from build123d import *

# Parameters (mm, degrees)
SKETCH_W        = 50
SKETCH_H        = 30
SKETCH_R        = 1.7
PAD_DEPTH       = 30
SKETCH001_W     = 16
SKETCH001_H     = 35
POCKET_DEPTH    = 24
POCKET001_DEPTH = 4
SKETCH003_R     = 2.5
POCKET002_DEPTH = 1.7
SKETCH004_R     = 3.6
POCKET003_DEPTH = 24
POCKET004_DEPTH = 4
SKETCH006_R     = 1.5
POCKET005_DEPTH = 20
FILLET_R        = 4
FILLET001_R     = 4
FILLET002_R     = 4
FILLET003_R     = 4
FILLET004_R     = 1
FILLET005_R     = 1
FILLET006_R     = 1
FILLET007_R     = 1
FILLET008_R     = 1
FILLET009_R     = 1
FILLET010_R     = 1
FILLET011_R     = 1


with BuildPart() as part:
    # Sketch → Pad (new body)
    with BuildSketch(Plane.XY):
        Rectangle(SKETCH_W, SKETCH_H)
        with Locations((18, 10)):
            Circle(SKETCH_R, mode=Mode.SUBTRACT)
        with Locations((18, -10)):
            Circle(SKETCH_R, mode=Mode.SUBTRACT)
        with Locations((-18, -10)):
            Circle(SKETCH_R, mode=Mode.SUBTRACT)
        with Locations((-18, 10)):
            Circle(SKETCH_R, mode=Mode.SUBTRACT)
    extrude(amount=PAD_DEPTH)

    # Sketch001 → Pocket (cut)
    with BuildSketch(Plane.XY.offset(30)):
        with Locations((-10, 0)):
            Rectangle(SKETCH001_W, SKETCH001_H)
        with Locations((10, 0)):
            Rectangle(SKETCH001_W, SKETCH001_H)
    extrude(amount=-POCKET_DEPTH, mode=Mode.SUBTRACT)

    # Sketch002 → Pocket001 (cut)
    with BuildSketch(Plane(origin=(0, 0, 0), x_dir=(1, 0, 0), z_dir=(0, 0, -1))):
        Polygon((-12.309401, 4), (-14.618802, 0), (-12.309401, -4), (-7.690599, -4), (-5.381198, 0), (-7.690599, 4), align=None)
        Polygon((7.690599, 4), (5.381198, 0), (7.690599, -4), (12.309401, -4), (14.618802, 0), (12.309401, 4), align=None)
    extrude(amount=-POCKET001_DEPTH, mode=Mode.SUBTRACT)

    # Sketch003 → Pocket002 (cut)
    with BuildSketch(Plane.XY.offset(6)):
        with Locations((-10, 0)):
            Circle(SKETCH003_R)
        with Locations((10, 0)):
            Circle(SKETCH003_R)
    extrude(amount=-POCKET002_DEPTH, mode=Mode.SUBTRACT)

    # Sketch004 → Pocket003 (cut)
    with BuildSketch(Plane.XY.offset(30)):
        with Locations((-18, 10)):
            Circle(SKETCH004_R)
        with Locations((18, 10)):
            Circle(SKETCH004_R)
        with Locations((-18, -10)):
            Circle(SKETCH004_R)
        with Locations((18.251301, -10.165039)):
            Circle(SKETCH004_R)
    extrude(amount=-POCKET003_DEPTH, mode=Mode.SUBTRACT)

    # Sketch005 → Pocket004 (cut)
    with BuildSketch(Plane.XY.offset(6)):
        Polygon((-19.558846, 12.7), (-21.117691, 10), (-19.558846, 7.3), (-16.441154, 7.3), (-14.882309, 10), (-16.441154, 12.7), align=None)
        Polygon((16.441154, 12.7), (14.882309, 10), (16.441154, 7.3), (19.558846, 7.3), (21.117691, 10), (19.558846, 12.7), align=None)
        Polygon((16.441154, -7.3), (14.882309, -10), (16.441154, -12.7), (19.558846, -12.7), (21.117691, -10), (19.558846, -7.3), align=None)
        Polygon((-21.117691, -10), (-19.558846, -12.7), (-16.441154, -12.7), (-14.882309, -10), (-16.441154, -7.3), (-19.558846, -7.3), align=None)
    extrude(amount=-POCKET004_DEPTH, mode=Mode.SUBTRACT)

    # Sketch006 → Pocket005 (cut)
    with BuildSketch(Plane.XY.offset(30)):
        with Locations((-21, 0)):
            Circle(SKETCH006_R)
        with Locations((21, 0)):
            Circle(SKETCH006_R)
    extrude(amount=-POCKET005_DEPTH, mode=Mode.SUBTRACT)

    # Fillet
    fillet_edges = [part.edges().sort_by_distance(p)[0] for p in [
        (-25, -15, 15),
    ]]
    fillet(fillet_edges, radius=FILLET_R)

    # Fillet001
    fillet001_edges = [part.edges().sort_by_distance(p)[0] for p in [
        (25, -15, 15),
    ]]
    fillet(fillet001_edges, radius=FILLET001_R)

    # Fillet002
    fillet002_edges = [part.edges().sort_by_distance(p)[0] for p in [
        (25, 15, 15),
    ]]
    fillet(fillet002_edges, radius=FILLET002_R)

    # Fillet003
    fillet003_edges = [part.edges().sort_by_distance(p)[0] for p in [
        (-25, 15, 15),
    ]]
    fillet(fillet003_edges, radius=FILLET003_R)

    # Fillet004
    fillet004_edges = [part.edges().sort_by_distance(p)[0] for p in [
        (-2, -15, 18),
    ]]
    fillet(fillet004_edges, radius=FILLET004_R)

    # Fillet005
    fillet005_edges = [part.edges().sort_by_distance(p)[0] for p in [
        (2, -15, 18),
    ]]
    fillet(fillet005_edges, radius=FILLET005_R)

    # Fillet006
    fillet006_edges = [part.edges().sort_by_distance(p)[0] for p in [
        (-2, 15, 18),
    ]]
    fillet(fillet006_edges, radius=FILLET006_R)

    # Fillet007
    fillet007_edges = [part.edges().sort_by_distance(p)[0] for p in [
        (2, 15, 18),
    ]]
    fillet(fillet007_edges, radius=FILLET007_R)

    # Fillet008
    fillet008_edges = [part.edges().sort_by_distance(p)[0] for p in [
        (18, 15, 18),
    ]]
    fillet(fillet008_edges, radius=FILLET008_R)

    # Fillet009
    fillet009_edges = [part.edges().sort_by_distance(p)[0] for p in [
        (-18, 15, 18),
    ]]
    fillet(fillet009_edges, radius=FILLET009_R)

    # Fillet010
    fillet010_edges = [part.edges().sort_by_distance(p)[0] for p in [
        (-18, -15, 18),
    ]]
    fillet(fillet010_edges, radius=FILLET010_R)

    # Fillet011
    fillet011_edges = [part.edges().sort_by_distance(p)[0] for p in [
        (18, -15, 18),
    ]]
    fillet(fillet011_edges, radius=FILLET011_R)


solid = part.part
Verification items for the finished model (mm, model axes). A direction names the side the tool comes from. Give positions to 0.01 mm unless a question says otherwise; leave off trailing zeros. Write each loop counter-clockwise with the first axis right and the second up, starting at its lowest first coordinate (ties: lowest second). Pieces come first, ordered by that corner, then holes.
(1) Material ranges on line 1 (X direction, y = -10, z = 1.5); line 2 (X direction, y = 1.75, z = 20.5); line 3 (Y direction, x = -18, z = 0.55), recorded low to high.
(2) Cross-section at B-B (x = -10). Enter the section's corners in (y, z), plus the area to 4 significant figures.
(3) Cross-section at C-C (x = 6.5). Enter the section's corners in (y, z), plus the area to 3 significant figures.
(4) Gauge pin test, flat ends, axial feed: pin 1 (4.5 mm diameter, centred on x = -10, y = 0, fed in from +Z); pin 2 (1.5 mm diameter, centred on x = -20.5, y = 0.5, fed in from +Z); pin 3 (6.5 mm diameter, centred on x = 10, y = 0, fed in from +Z). Record the tip position at first contact, or that the pin passes through.
(5) Cross-section at D-D (x = -4). Enter the section's corners in (y, z), plus the area to 3 significant figures.
(6) Cross-section at A-A (z = 24.5). State how many separate pieces and enclosed holes the cut face has, plus the area to 3 significant figures.
(7) Access from +Z, -Z, +X, -X, +Y, -Y to the whole of each face (thin tool, end or side, straight path). Record for faces 1 (the face through (-1.715, 14.699, 17.832)), 2 (the face through (-15.65, 11.33, 4.03)), 3 (the face through (10, 4, 2)), 4 (the face through (18.285, -14.699, 17.832)).
(8) Mould release check, pull along X, two halves, no side actions. Record for faces 5 (the face through (-18, 12, 2)), 6 (the face through (0, 15, 7)): +X half, -X half, draft (parallel to the pull), parting line (faces both ways), or undercut.
Worked out:
1. line 1: x = -25 to -19.7, -16.3 to 16.3, 19.7 to 25
1. line 2: x = -25 to -18, -2 to 2, 18 to 25
1. line 3: y = -15 to -11.7, -8.3 to 8.3, 11.7 to 15
2. outline: (-15, 0) - (-4, 0) - (-4, 4) - (4, 4) - (4, 0) - (15, 0) - (15, 6) - (2.5, 6) - (2.5, 4.3) - (-2.5, 4.3) - (-2.5, 6) - (-15, 6) - close
2. area: 139.5 mm2
3. outline: (-15, 0) - (-1.94, 0) - (-1.94, 4) - (1.94, 4) - (1.94, 0) - (15, 0) - (15, 6) - (-15, 6) - close
3. area: 164 mm2
4. pin 1: stops at z = 4.3
4. pin 2: stops at z = 10
4. pin 3: stops at z = 6
5. outline: (-15, 0) - (15, 0) - (15, 6) - (-15, 6) - close
5. area: 180 mm2
6. separate pieces: 3
6. enclosed holes: 2
6. area: 427 mm2
7. face 1: +Z, +Y
7. face 2: +Z
7. face 3: -Z
7. face 4: +Z, -Y
8. face 5: undercut
8. face 6: draft
